Could you check a few things on this drawing? It's one solid part, dimensions in mm from its lowest x, y, z. A direction names the side the tool comes from. Give positions to 0.01 mm unless a question says otherwise; leave off trailing zeros. Order: outer loops, then holes, each group sorted by start corner. A loop starts at its lowest first (then second) coordinate and runs counter-clockwise, first axis right, second up.
(1) On a 3-axis mill with a long thin cutter (end or side, diameter ignored), from which of +Z, -Z, +X, -X, +Y, -Y can I reach the whole of each face in a straight line? I mean the marked faces 1 and 2. Say none if no direction works.
(2) Imagine slicing it at B-B, the plane y = 24. Write out the boundary of the cut face in (x, z) (1 decimal), then the cut area to 3 significant figures.
(3) Imagine slicing it at D-D, the plane y = 146. Write out the boundary of the cut face in (x, z) (1 decimal).
(4) Will these pins go through, and if not, where does the flat tip stop? pin 1 (2 mm diameter, centred on y = 178, z = 4.5, fed in from +X); pin 2 (2 mm diameter, centred on x = 99.5, z = 15, fed in from +Y); pin 3 (8 mm diameter, centred on y = 92, z = 12, fed in from -X); pin 4 (10 mm diameter, centred on x = 104.5, y = 146, fed in from -Z).
(5) Imagine slicing it at A-A, the plane z = 13.75. Write out the boundary of the cut face in (x, y) (1 decimal).
(6) Imagine slicing it at C-C, the plane x = 81.5. Write out the boundary of the cut face in (y, z) (1 decimal).
(7) If we mould it in two halves opening along X, with no side actions, what happens to the marked faces 3, 4 and 5? For each: released by +X, released by -X, zero draft, split by the parting line, or undercut.
(8) If I drill on probe 1 along X at (y, z) = (126.5, 6) (1 decimal); probe 2 along X at (y, z) = (75.5, 1.75) (1 decimal); probe 3 along X at (y, z) = (140, 16.5) (1 decimal), over which ranges is the centre line in solid material (lowest first)?
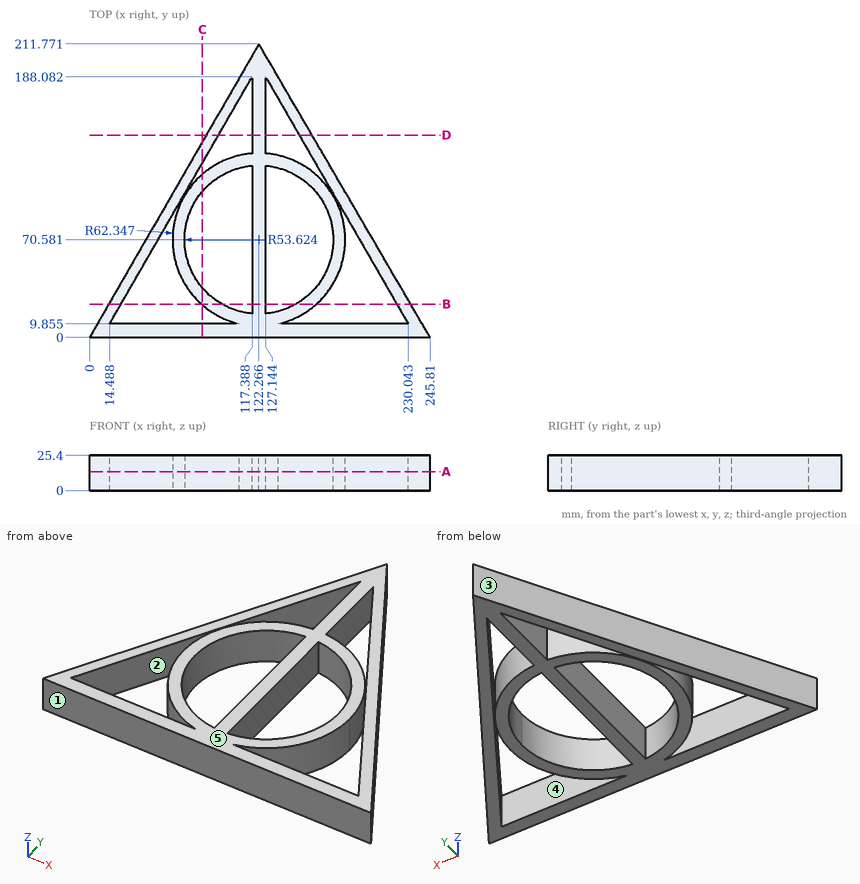
Answer block:
1. face 1: +Z, -Z, +X, -X, -Y
1. face 2: +Z, -Z
2. outline: (13.9, 0) - (22.7, 0) - (22.7, 25.4) - (13.9, 25.4) - close; (80.8, 0) - (95.7, 0) - (95.7, 25.4) - (80.8, 25.4) - close; (117.4, 0) - (127.1, 0) - (127.1, 25.4) - (117.4, 25.4) - close; (148.8, 0) - (163.7, 0) - (163.7, 25.4) - (148.8, 25.4) - close; (221.9, 0) - (231.8, 0) - (231.8, 25.4) - (221.9, 25.4) - close
2. area: 1,480 mm2
3. outline: (84.3, 0) - (93.1, 0) - (93.1, 25.4) - (84.3, 25.4) - close; (117.4, 0) - (127.1, 0) - (127.1, 25.4) - (117.4, 25.4) - close; (151.4, 0) - (160.6, 0) - (160.6, 25.4) - (151.4, 25.4) - close
4. pin 1: stops at x = 142.55
4. pin 2: stops at y = 174.07
4. pin 3: stops at x = 50.81
4. pin 4: passes through
5. outline: (0, 0) - (245.8, 0) - (122.3, 211.8) - close; hole (14.5, 9.9) - (108.1, 9.9) arc R62.3 cw to (117.4, 132.7) - (117.4, 188.1) - close; hole (117.4, 17.2) - (117.4, 124) arc R53.6 ccw to start; hole (127.1, 17.2) arc R53.6 ccw to (127.1, 124) - close; hole (127.1, 132.7) arc R62.3 cw to (136.4, 9.9) - (230, 9.9) - (127.1, 188.1) - close
6. outline: (0, 0) - (9.9, 0) - (9.9, 25.4) - (0, 25.4) - close; (23.4, 0) - (35.7, 0) - (35.7, 25.4) - (23.4, 25.4) - close; (105.4, 0) - (117.8, 0) - (117.8, 25.4) - (105.4, 25.4) - close; (125.9, 0) - (141.2, 0) - (141.2, 25.4) - (125.9, 25.4) - close
7. face 3: released by -X
7. face 4: undercut
7. face 5: zero draft
8. probe 1: x = 73 to 81.8, 94.7 to 149.8, 162.7 to 172
8. probe 2: x = 43.6 to 52.4, 60.1 to 68.9, 117.4 to 127.1, 175.7 to 184.4, 192.1 to 201.8
8. probe 3: x = 80.8 to 89.6, 117.4 to 127.1, 154.9 to 164.1
